Could you check a few things on this model? Use its own coordinates, in mm. A direction names the side the tool comes from. Round coordinates to 2 decimals unless told otherwise and drop trailing zeros. Loops run counter-clockwise (first coordinate to the right, second up) from the corner with the lowest first, then second, coordinate; pieces in that order, holes last. Notation, with made-up numbers: (74.25, 44) - (99.25, 44) arc R27 cw to (99.25, 71) - close; hole circle Ø6 at (87, -4). An arc over 180 degrees is marked (long way). Use one line per item in the form item = value.
```python
from build123d import *

# Parameters (mm, degrees)
SKETCH1_R           = 30
SKETCH1_R_2         = 16
BOSS_EXTRUDE1_DEPTH = 25
BOSS_EXTRUDE5_DEPTH = 7.5
BOSS_EXTRUDE6_DEPTH = 50
SKETCH7_3_R         = 10
BOSS_EXTRUDE7_DEPTH = 12.5


with BuildPart() as part:
    # Sketch1 → Boss-Extrude1 (new, symmetric)
    with BuildSketch(Plane.XY):
        Circle(SKETCH1_R)
        Circle(SKETCH1_R_2, mode=Mode.SUBTRACT)
    extrude(amount=BOSS_EXTRUDE1_DEPTH, both=True)

    # Sketch2 → Boss-Extrude5 (add, symmetric)
    with BuildSketch(Plane.XY):
        with BuildLine():
            ThreePointArc((-30, 0), (-21.213203436, 21.213203436), (0, 30))
            Line((0, 30), (0, 40))
            Line((0, 40), (-30, 40))
            Line((-30, 40), (-30, 0))
        make_face()
        with BuildLine():
            Line((0, 40), (0, 30))
            ThreePointArc((0, 30), (21.213203436, 21.213203436), (30, 0))
            Line((30, 0), (30, 40))
            Line((30, 40), (0, 40))
        make_face()
    extrude(amount=BOSS_EXTRUDE5_DEPTH, both=True)

    # Sketch7 → Boss-Extrude6 (add)
    with BuildSketch(Plane.XY.offset(25)):
        Polygon((-30, 40), (0, 40), (0, 55), (-26.456439237, 55), align=None)
        Polygon((0, 55), (0, 40), (30, 40), (26.456439237, 55), align=None)
    extrude(amount=-BOSS_EXTRUDE6_DEPTH)

    # Sketch7_3 → Boss-Extrude7 (add)
    with BuildSketch(Plane.XY.offset(25)):
        with BuildLine():
            Line((-30, 40), (30, 40))
            Line((30, 40), (19.464242224, 84.598181668))
            ThreePointArc((19.464242224, 84.598181668), (0, 100), (-19.464242224, 84.598181668))
            Line((-19.464242224, 84.598181668), (-30, 40))
        make_face()
        with Locations((0, 80)):
            Circle(SKETCH7_3_R, mode=Mode.SUBTRACT)
    boss_extrude7 = extrude(amount=-BOSS_EXTRUDE7_DEPTH)

    # Mirror2: Boss-Extrude7 across plane
    add(boss_extrude7.mirror(Plane.XY))


solid = part.part
```
1. Please list where these lines run through material, in increasing order: line 1 along Y through (x, z) = (0, 22); line 2 along Y through (x, z) = (0, 6); line 3 along Z through (x, y) = (13.5, 57).
Solution:
line_1 = -30 to -16, 16 to 30, 40 to 70, 90 to 100
line_2 = -30 to -16, 16 to 55
line_3 = -25 to -12.5, 12.5 to 25
2. If we section it at C-C, the plane y = 18: Write out the boundary of the cut face in (x, z).
Solution:
outline = (-30, -7.5) - (-24, -7.5) - (-24, -25) - (24, -25) - (24, -7.5) - (30, -7.5) - (30, 7.5) - (24, 7.5) - (24, 25) - (-24, 25) - (-24, 7.5) - (-30, 7.5) - close
3. If we section it at D-D, the plane x = 22.5: Write out the boundary of the cut face in (y, z), plus the area to 3 significant figures.
Solution:
outline = (-19.84, -25) - (19.84, -25) - (19.84, -7.5) - (40, -7.5) - (40, -25) - (71.75, -25) - (71.75, -12.5) - (55, -12.5) - (55, 12.5) - (71.75, 12.5) - (71.75, 25) - (40, 25) - (40, 7.5) - (19.84, 7.5) - (19.84, 25) - (-19.84, 25) - close
area = 3,460 mm^2
4. For P1, Ø12, axis at y = 20.5, z = 16.5, coming from the -X side; P2, Ø1.5, axis at x = -20.5, y = 35, coming from the +Z side; P3, Ø4, axis at x = -13, z = 13, coming from the -Y side; P4, Ø12, axis at x = 0, y = 80, coming from the -Z side, each with a flat end and sliding along its axis, tell me the tip position at first contact or that it passes through.
Solution:
P1 = -26.26
P2 = 7.5
P3 = -27.91
P4 = through
5. If we section it at A-A, the plane x = 0: Write out the boundary of the cut face in (y, z), plus the area to 4 significant figures.
Solution:
outline = (-30, -25) - (-16, -25) - (-16, 25) - (-30, 25) - close; (16, -25) - (30, -25) - (30, -7.5) - (40, -7.5) - (40, -25) - (70, -25) - (70, -12.5) - (55, -12.5) - (55, 12.5) - (70, 12.5) - (70, 25) - (40, 25) - (40, 7.5) - (30, 7.5) - (30, 25) - (16, 25) - close; (90, -25) - (100, -25) - (100, -12.5) - (90, -12.5) - close; (90, 12.5) - (100, 12.5) - (100, 25) - (90, 25) - close
area = 2,925 mm^2
6. We'd pull the mould along Z, two halves only. Please class faces 5 (the face through (0, 100, -19)), 6 (the face through (0, 68, 12.5)), 7 (the face through (13, -13, 25)): +Z half, -Z half, draft (parallel to the pull), parting line (faces both ways), or undercut.
Solution:
face_5 = draft
face_6 = undercut
face_7 = +Z half
7. On a 3-axis mill with a long thin cutter (end or side, diameter ignored), from which of +Z, -Z, +X, -X, +Y, -Y can I reach the whole of each face in a straight line? I mean faces 1 (the face through (0, 34, 7.5)), 2 (the face through (0, 40, -16)), 3 (the face through (0, 55, 0)), 4 (the face through (13.843, -26.615, 0.35)). Say none if no direction works.
Solution:
face_1 = +Z
face_2 = -Z, +X, -X
face_3 = +X, -X, +Y
face_4 = none
8. If we section it at B-B, the plane y = 71.5: Write out the boundary of the cut face in (x, z), plus the area to 3 significant figures.
Solution:
outline = (-22.56, -25) - (-5.27, -25) - (-5.27, -12.5) - (-22.56, -12.5) - close; (-22.56, 12.5) - (-5.27, 12.5) - (-5.27, 25) - (-22.56, 25) - close; (5.27, -25) - (22.56, -25) - (22.56, -12.5) - (5.27, -12.5) - close; (5.27, 12.5) - (22.56, 12.5) - (22.56, 25) - (5.27, 25) - close
area = 865 mm^2
